Can you work these out from the model? Positions are in its coordinate system, mm. A direction names the side the tool comes from. Give positions to 0.01 mm unless a question says otherwise; leave off trailing zeros. Order: outer loops, then holes, each group sorted by start corner. A loop starts at its lowest first (then second) coordinate and runs counter-clockwise, first axis right, second up. Notation, with made-up numbers: (10.25, -31) - (65.25, -31) arc R21 ccw to (65.25, -9) - close; hole circle Ø9 at (-27, 3.5). An arc over 180 degrees is marked (long way). Answer as a JSON object with one key per item and string values.
```python
from build123d import *

# Parameters (mm, degrees)
ESQUISSE1_W             = 26
ESQUISSE1_H             = 26
ESQUISSE1_R             = 10.6
BOSS_EXTRU_1_DEPTH      = 40.7
ESQUISSE7_W             = 26
ESQUISSE7_H             = 26
ESQUISSE7_R             = 7.5
BOSS_EXTRU_5_DEPTH      = 3
ESQUISSE9_W             = 11.7
ESQUISSE9_H             = 5
BOSS_EXTRU_6_DEPTH      = 5
ESQUISSE11_R            = 1.75
ENL_V_MAT_EXTRU_1_DEPTH = 52.717405194
ESQUISSE17_W            = 11.7
ESQUISSE17_H            = 5
BOSS_EXTRU_7_DEPTH      = 5
ESQUISSE18_R            = 1.75
ENL_V_MAT_EXTRU_2_DEPTH = 52.717405194


with BuildPart() as part:
    # Esquisse1 → Boss.-Extru.1 (new body)
    with BuildSketch(Plane.XY):
        with Locations((0, -2.19)):
            Rectangle(ESQUISSE1_W, ESQUISSE1_H)
        Circle(ESQUISSE1_R, mode=Mode.SUBTRACT)
    extrude(amount=BOSS_EXTRU_1_DEPTH)

    # Esquisse7 → Boss.-Extru.5 (add)
    with BuildSketch(Plane.XY.offset(40.7)):
        with Locations((0, -2.19)):
            Rectangle(ESQUISSE7_W, ESQUISSE7_H)
        Circle(ESQUISSE7_R, mode=Mode.SUBTRACT)
    extrude(amount=BOSS_EXTRU_5_DEPTH)

    # Esquisse9 → Boss.-Extru.6 (add)
    with BuildSketch(Plane.ZY.offset(13)):
        with Locations((21.85, -12.69)):
            Rectangle(ESQUISSE9_W, ESQUISSE9_H)
    extrude(amount=BOSS_EXTRU_6_DEPTH)

    # Esquisse11 → Enl_v. mat.-Extru.1 (cut, through all)
    with BuildSketch(Plane(origin=(0, -10.19, 0), x_dir=(1, 0, 0), z_dir=(0, 1, 0))):
        with Locations(Location((-15.450046311, -19, 0), (0, 0, 180))):
            Circle(ESQUISSE11_R)
        with Locations(Location((-15.450046311, -24.7, 0), (0, 0, 180))):
            Circle(ESQUISSE11_R)
    extrude(amount=-ENL_V_MAT_EXTRU_1_DEPTH, mode=Mode.SUBTRACT)

    # Esquisse17 → Boss.-Extru.7 (add)
    with BuildSketch(Plane(origin=(13, 0, 0), x_dir=(0, 0, -1), z_dir=(1, 0, 0))):
        with Locations((-21.85, -12.69)):
            Rectangle(ESQUISSE17_W, ESQUISSE17_H)
    extrude(amount=BOSS_EXTRU_7_DEPTH)

    # Esquisse18 → Enl_v. mat.-Extru.2 (cut, through all)
    with BuildSketch(Plane(origin=(0, -10.19, 0), x_dir=(1, 0, 0), z_dir=(0, 1, 0))):
        with Locations(Location((15.5, -24.7, 0), (0, 0, 180))):
            Circle(ESQUISSE18_R)
        with Locations(Location((15.5, -19, 0), (0, 0, 180))):
            Circle(ESQUISSE18_R)
    extrude(amount=-ENL_V_MAT_EXTRU_2_DEPTH, mode=Mode.SUBTRACT)


solid = part.part
```
Q1. I need wall thicknesses on L1, parallel to Z at x = 15.5, y = -11.15; L2, parallel to X at y = -7.5, z = 22; L3, parallel to Y at x = 0, z = 42.65. Which ranges of each line are inside material? Lowest first, please.
Recorded:
{"L1": "z = 16 to 17.25, 20.75 to 22.95, 26.45 to 27.7", "L2": "x = -13 to -7.49, 7.49 to 13", "L3": "y = -15.19 to -7.5, 7.5 to 10.81"}
Q2. If we section it at B-B, the plane z = 19: Please give me the cut outline in (x, y), then the cut area to 3 significant figures.
Recorded:
{"outline": "(-18, -15.19) - (-17.2, -15.19) - (-17.2, -10.19) - (-18, -10.19) - close; (-13.7, -15.19) - (13.75, -15.19) - (13.75, -10.19) - (13, -10.19) - (13, 10.81) - (-13, 10.81) - (-13, -10.19) - (-13.7, -10.19) - close; (17.25, -15.19) - (18, -15.19) - (18, -10.19) - (17.25, -10.19) - close; hole circle Ø21.2 at (0, 0)", "area": "338 mm^2"}
Q3. We'd pull the mould along Z, two halves only. Please class faces 1 (the face through (0, -8, 43.7)), 2 (the face through (-7.493, 0.33, 42.179)), 3 (the face through (15.728, -12.655, 20.735)): released by +Z, released by -Z, zero draft, split by the parting line, or undercut.
Recorded:
{"face 1": "released by +Z", "face 2": "zero draft", "face 3": "undercut"}
Q4. I'm going to push flat-ended pins straight in: pin 1 Ø1.5 at (x, z) = (16.5, 19.5) entering from +Y; pin 2 Ø1.5 at (x, y) = (-16, -12) entering from -Z; pin 3 Ø5.5 at (x, y) = (16, -14) entering from +Z; pin 4 Ø2 at (x, z) = (15.5, 24.7) entering from +Y. Where does each tip first touch, or does it pass through?
Recorded:
{"pin 1": "stops at y = -10.19", "pin 2": "stops at z = 16", "pin 3": "stops at z = 27.7", "pin 4": "passes through"}
Q5. Which directions (+Z, -Z, +X, -X, +Y, -Y) give clear straight access to the entire face, cutting with the end or side of a thin tool? Please do faces 4 (the face through (-15, -10.19, 22)), 5 (the face through (15, -10.19, 22)), 6 (the face through (5, -7, 40.7)), 7 (the face through (15, -13, 16)), 8 (the face through (15, -13, 27.7)).
Recorded:
{"face 4": "+Z, -Z, -X, +Y", "face 5": "+Z, -Z, +X, +Y", "face 6": "-Z", "face 7": "-Z, +X, +Y, -Y", "face 8": "+Z, +X, +Y, -Y"}
Q6. If we section it at A-A, the plane x = 15.5: Please give me the cut outline in (y, z), then the cut area to 3 significant figures.
Recorded:
{"outline": "(-15.19, 16) - (-10.19, 16) - (-10.19, 17.25) - (-15.19, 17.25) - close; (-15.19, 20.75) - (-10.19, 20.75) - (-10.19, 22.95) - (-15.19, 22.95) - close; (-15.19, 26.45) - (-10.19, 26.45) - (-10.19, 27.7) - (-15.19, 27.7) - close", "area": "23.5 mm^2"}
Q7. If we section it at D-D, the plane x = 0: Please give me the cut outline in (y, z).
Recorded:
{"outline": "(-15.19, 0) - (-10.6, 0) - (-10.6, 40.7) - (-7.5, 40.7) - (-7.5, 43.7) - (-15.19, 43.7) - close; (7.5, 40.7) - (10.6, 40.7) - (10.6, 0) - (10.81, 0) - (10.81, 43.7) - (7.5, 43.7) - close"}
Q8. If we section it at C-C, the plane y = -11.5: Please give me the cut outline in (x, z).
Recorded:
{"outline": "(-18, 16) - (-13, 16) - (-13, 0) - (13, 0) - (13, 16) - (18, 16) - (18, 27.7) - (13, 27.7) - (13, 43.7) - (-13, 43.7) - (-13, 27.7) - (-18, 27.7) - close; hole circle Ø3.5 at (-15.45, 19); hole circle Ø3.5 at (-15.45, 24.7); hole circle Ø3.5 at (15.5, 19); hole circle Ø3.5 at (15.5, 24.7)"}
